The listing builds one solid part. Answer for the finished solid, in the listing's coordinates (mm). A direction names the side the tool comes from. Give positions to 0.01 mm unless a question says otherwise; leave off trailing zeros. Loops run counter-clockwise (first coordinate to the right, second up) from the corner with the lowest first, then second, coordinate; pieces in that order, holes last. Notation, with made-up numbers: (6.5, -9.75) -> (36.5, -9.75) arc R23 ccw to (36.5, 1.25) -> close; hole circle Ø9 at (84.5, 88). An arc over 180 degrees is marked (long way). One line per question, with ' | ' between items. Start each with the question number.
from build123d import *

# Parameters (mm, degrees)
IZIM1_W                     = 46
IZIM1_H                     = 18.5
Y_KSEKLIK_EKSTR_ZYON1_DEPTH = 30.95
IZIM2_W                     = 46
IZIM2_H                     = 14.5
KES_EKSTR_ZYON1_DEPTH       = 3.15
IZIM3_W                     = 46
IZIM3_H                     = 2
Y_KSEKLIK_EKSTR_ZYON2_DEPTH = 2
IZIM4_W                     = 46
IZIM4_H                     = 2
Y_KSEKLIK_EKSTR_ZYON3_DEPTH = 2


with BuildPart() as part:
    # Çizim1 → Yükseklik-Ekstrüzyon1 (new body)
    with BuildSketch(Plane.XY):
        Rectangle(IZIM1_W, IZIM1_H)
    extrude(amount=-Y_KSEKLIK_EKSTR_ZYON1_DEPTH)

    # Çizim2 → Kes-Ekstrüzyon1 (cut)
    with BuildSketch(Plane(origin=(0, 0, -30.95), x_dir=(-1, 0, 0), z_dir=(0, 0, -1))):
        Rectangle(IZIM2_W, IZIM2_H)
    extrude(amount=-KES_EKSTR_ZYON1_DEPTH, mode=Mode.SUBTRACT)

    # Çizim3 → Yükseklik-Ekstrüzyon2 (add)
    with BuildSketch(Plane.XZ.offset(9.25)):
        with Locations((0, -1)):
            Rectangle(IZIM3_W, IZIM3_H)
    extrude(amount=Y_KSEKLIK_EKSTR_ZYON2_DEPTH)

    # Çizim4 → Yükseklik-Ekstrüzyon3 (add)
    with BuildSketch(Plane(origin=(0, 9.25, 0), x_dir=(1, 0, 0), z_dir=(0, 1, 0))):
        with Locations((0, 1)):
            Rectangle(IZIM4_W, IZIM4_H)
    extrude(amount=Y_KSEKLIK_EKSTR_ZYON3_DEPTH)


solid = part.part
1. The part is cut by section B-B (y = -6.75). Write down the section's boundary in (x, z), plus the area to 3 significant figures.
2. The part is cut by section A-A (x = -18). Write down the section's boundary in (y, z).
3. Straight lines are drawn through the part: L1, parallel to Y at x = 12, z = -29; L2, parallel to Y at x = 5, z = -21; L3, parallel to Z at x = 19.5, y = -5. For each, find the intervals that lie inside material, in ascending order.
4. The part is cut by section C-C (z = -8). Write down the section's boundary in (x, y), plus the area to 3 significant figures.
5. For faces 4 (the flat face through (0, -11.25, -1)), 5 (the flat face through (0, -10, -2)), 6 (the flat face through (-23, 0, -15)), 7 (the flat face through (0, 7.25, -29)), 8 (the flat face through (0, 9.25, -16)), determine the directions among +Z, -Z, +X, -X, +Y, -Y from which every point of the face is accessible in a straight line to the end or side of a thin tool.
6. Determine the mould class of faces 1 (the flat face through (0, -9.25, -16)), 2 (the flat face through (0, -7.25, -29)), 3 (the flat face through (0, -8, -30.95)) for opening direction Y: released by +Y, released by -Y, zero draft, split by the parting line, or undercut.
7. Each of these flat-tipped pins is pushed along its axis until it touches: pin 1 Ø4.5 at (x, y) = (4, -2) entering from -Z; pin 2 Ø1 at (x, y) = (-1.5, 10.5) entering from -Z; pin 3 Ø3 at (x, z) = (12.5, -16.5) entering from +Y. Where does it stop, or does it pass through?
Check sheet entries:
1) outline: (-23, -27.8) -> (23, -27.8) -> (23, 0) -> (-23, 0) -> close | area: 1,280 mm^2
2) outline: (-11.25, -2) -> (-9.25, -2) -> (-9.25, -30.95) -> (-7.25, -30.95) -> (-7.25, -27.8) -> (7.25, -27.8) -> (7.25, -30.95) -> (9.25, -30.95) -> (9.25, -2) -> (11.25, -2) -> (11.25, 0) -> (-11.25, 0) -> close
3) L1: y = -9.25 to -7.25, 7.25 to 9.25 | L2: y = -9.25 to 9.25 | L3: z = -27.8 to 0
4) outline: (-23, -9.25) -> (23, -9.25) -> (23, 9.25) -> (-23, 9.25) -> close | area: 851 mm^2
5) face 4: +Z, -Z, +X, -X, -Y | face 5: -Z, +X, -X, -Y | face 6: +Z, -Z, -X, +Y, -Y | face 7: -Z, +X, -X | face 8: -Z, +X, -X, +Y
6) face 1: released by -Y | face 2: undercut | face 3: zero draft
7) pin 1: stops at z = -27.8 | pin 2: stops at z = -2 | pin 3: stops at y = 9.25
